CAD build for the part. Positions are in the model's coordinates, mm. Round coordinates to 2 decimals unless told otherwise and drop trailing zeros. Loops run counter-clockwise (first coordinate to the right, second up) from the corner with the lowest first, then second, coordinate; pieces in that order, holes last. Notation, with made-up numbers: M -13,22 L 12,22 A10 ccw 12,29 Z; hole C 66,12.5 d10. An arc over 180 degrees is marked long. Use one line per item in the form item = value.
Autodesk Inventor part; units mm, degrees
ref_plane "YZ Plane" through (0, 0, 0) normal (1, 0, 0) x (0, 1, 0)
ref_plane "XZ Plane" through (0, 0, 0) normal (0, 1, 0) x (-1, 0, 0)
ref_plane "XY Plane" through (0, 0, 0) normal (0, 0, 1) x (1, 0, 0)
sketch "Sketch1" plane through (0, 0, 0) normal (1, 0, 0) x (0, 1, 0)
  line L0 (0, 0) -> (25.4, 0)
  line L1 (25.4, 0) -> (25.4, -254)
  line L2 (25.4, -254) -> (0, -254)
  line L3 (0, -254) -> (0, 0)
  dimension "d0" = 25.4
  dimension "d1" = 254
extrude "Extrusion1" add sketch "Sketch1" along normal blind 3.175
hole "Hole1" at (3.175, 12.7, -241.3) direction (-1, 0, 0) diameter 5.1594 end through all
properties part number "0.125 in Flatbar Support Beam"
1. Cut at B-B on z = -241.3. Write the cut outline in (x, y) (3 decimals), and give its area (3 significant figures).
Completed:
outline = M 0,0 L 3.175,0 L 3.175,10.12 L 0,10.12 Z; M 0,15.28 L 3.175,15.28 L 3.175,25.4 L 0,25.4 Z
area = 64.3 mm2
2. Pull direction Y, two halves, no side cores. Call faces 1 (the face through (1.565, 13.688, -243.683)), 2 (the face through (3.175, 13, -125)): +Y half, -Y half, draft (parallel to the pull), parting line (faces both ways), or undercut.
Completed:
face_1 = undercut
face_2 = draft
3. Probe line 1 along Z through (x, y) = (2.05, 12.7); line 2 along Y through (x, z) = (0.6, -241.3); line 3 along Z through (x, y) = (0.25, 11.25). List the from-to ranges inside material, lowest first. Write a range as from..to.
Completed:
line_1 = -254..-243.88, -238.72..0
line_2 = 0..10.12, 15.28..25.4
line_3 = -254..-243.43, -239.17..0
4. Cut at A-A on y = 12.7. Write the cut outline in (x, z) (3 decimals).
Completed:
outline = M 0,-254 L 3.175,-254 L 3.175,-243.88 L 0,-243.88 Z; M 0,-238.72 L 3.175,-238.72 L 3.175,0 L 0,0 Z
